```python
from build123d import *

# Parameters (mm, degrees)
BOX007_W          = 10
BOX007_H          = 10
BOX007_DEPTH      = 17
CYLINDER002_R     = 3.4
CYLINDER002_DEPTH = 13
BOX006_W          = 6
BOX006_H          = 10
BOX006_DEPTH      = 15
BOX005_W          = 6
BOX005_H          = 10
BOX005_DEPTH      = 15
CYLINDER001_R     = 15
CYLINDER001_DEPTH = 2.5
BOX004_W          = 6
BOX004_H          = 10
BOX004_DEPTH      = 15
BOX003_W          = 6
BOX003_H          = 10
BOX003_DEPTH      = 15
BOX002_W          = 6
BOX002_H          = 35
BOX002_DEPTH      = 10
BOX001_W          = 15
BOX001_H          = 35
BOX001_DEPTH      = 10
BOX_W             = 15
BOX_H             = 35
BOX_DEPTH         = 10
CYLINDER_R        = 15
CYLINDER_DEPTH    = 12
FILLET_R          = 4
FILLET001_R       = 1.5
FILLET002_R       = 1.5


with BuildPart() as cubo005:
    # Box007 → Box007 (new body)
    with BuildSketch(Plane(origin=(-5, 2.6, -28), x_dir=(1, 0, 0), z_dir=(0, 0, 1))):
        with Locations((5, 5)):
            Rectangle(BOX007_W, BOX007_H)
    extrude(amount=BOX007_DEPTH)


with BuildPart() as cut007:
    # Cylinder002 → Cylinder002 (new body)
    with BuildSketch(Plane.XY.offset(-26)):
        Circle(CYLINDER002_R)
    extrude(amount=CYLINDER002_DEPTH)

    # Cut007: cut Cubo005
    add(cubo005.part, mode=Mode.SUBTRACT)


with BuildPart() as cut007_1:
    # Cut007 placement: moved
    add(cut007.part.moved(Location((0, 0, 23))))


with BuildPart() as cubo004:
    # Box006 → Box006 (new body)
    with BuildSketch(Plane(origin=(-3, 14.4, -2), x_dir=(1, 0, 0), z_dir=(0, 0, 1))):
        with Locations((3, 5)):
            Rectangle(BOX006_W, BOX006_H)
    extrude(amount=BOX006_DEPTH)


with BuildPart() as cubo003:
    # Box005 → Box005 (new body)
    with BuildSketch(Plane(origin=(-3, -24.4, -2), x_dir=(1, 0, 0), z_dir=(0, 0, 1))):
        with Locations((3, 5)):
            Rectangle(BOX005_W, BOX005_H)
    extrude(amount=BOX005_DEPTH)


with BuildPart() as cilindro001:
    # Cylinder001 → Cylinder001 (new body)
    with BuildSketch(Plane.XY.offset(-2)):
        Circle(CYLINDER001_R)
    extrude(amount=CYLINDER001_DEPTH)


with BuildPart() as cubo002:
    # Box004 → Box004 (new body)
    with BuildSketch(Plane(origin=(-3, -24.4, -2), x_dir=(1, 0, 0), z_dir=(0, 0, 1))):
        with Locations((3, 5)):
            Rectangle(BOX004_W, BOX004_H)
    extrude(amount=BOX004_DEPTH)


with BuildPart() as cubo001:
    # Box003 → Box003 (new body)
    with BuildSketch(Plane(origin=(-3, 14.4, -2), x_dir=(1, 0, 0), z_dir=(0, 0, 1))):
        with Locations((3, 5)):
            Rectangle(BOX003_W, BOX003_H)
    extrude(amount=BOX003_DEPTH)


with BuildPart() as cubo:
    # Box002 → Box002 (new body)
    with BuildSketch(Plane(origin=(-3, -17, 11.7), x_dir=(1, 0, 0), z_dir=(0, 0, 1))):
        with Locations((3, 17.5)):
            Rectangle(BOX002_W, BOX002_H)
    extrude(amount=BOX002_DEPTH)


with BuildPart() as box001:
    # Box001 → Box001 (new body)
    with BuildSketch(Plane(origin=(-20, -15, 3), x_dir=(1, 0, 0), z_dir=(0, 0, 1))):
        with Locations((7.5, 17.5)):
            Rectangle(BOX001_W, BOX001_H)
    extrude(amount=BOX001_DEPTH)


with BuildPart() as box:
    # Box → Box (new body)
    with BuildSketch(Plane(origin=(5, -15, 3), x_dir=(1, 0, 0), z_dir=(0, 0, 1))):
        with Locations((7.5, 17.5)):
            Rectangle(BOX_W, BOX_H)
    extrude(amount=BOX_DEPTH)


with BuildPart() as fuel_knob:
    # Cylinder → Cylinder (new body)
    with BuildSketch(Plane.XY):
        Circle(CYLINDER_R)
    extrude(amount=CYLINDER_DEPTH)

    # Cut: cut Box
    add(box.part, mode=Mode.SUBTRACT)

    # Cut001: cut Box001
    add(box001.part, mode=Mode.SUBTRACT)

    # Cut002: cut Cubo
    add(cubo.part, mode=Mode.SUBTRACT)

    # Cut003: cut Cubo001
    add(cubo001.part, mode=Mode.SUBTRACT)

    # Cut004: cut Cubo002
    add(cubo002.part, mode=Mode.SUBTRACT)

    # Fusion: union Cilindro001
    add(cilindro001.part)

    # Cut005: cut Cubo003
    add(cubo003.part, mode=Mode.SUBTRACT)

    # Cut006: cut Cubo004
    add(cubo004.part, mode=Mode.SUBTRACT)

    # Fillet
    fillet_edges = [fuel_knob.edges().sort_by_distance(p)[0] for p in [
        (0, -14.4, 11.7),
        (0, 14.4, 11.7),
        (-4.009607, -14.454171, 12),
        (-4.009607, 14.454171, 12),
        (4.009607, 14.454171, 12),
        (4.009607, -14.454171, 12),
    ]]
    fillet(fillet_edges, radius=FILLET_R)

    # Fillet001
    fillet001_edges = [fuel_knob.edges().sort_by_distance(p)[0] for p in [
        (-5, 0, 3),
        (5, 0, 3),
    ]]
    fillet(fillet001_edges, radius=FILLET001_R)

    # Fillet002
    fillet002_edges = [fuel_knob.edges().sort_by_distance(p)[0] for p in [
        (-5, 0, 12),
        (5, 0, 12),
    ]]
    fillet(fillet002_edges, radius=FILLET002_R)

    # Cut008: cut Cut007
    add(cut007_1.part, mode=Mode.SUBTRACT)


solid = fuel_knob.part
```
Input: part model. Units: mm. Frame: model coordinates. A direction names the side the tool comes from. Give positions to 0.01 mm unless a question says otherwise; leave off trailing zeros. Write each loop counter-clockwise with the first axis right and the second up, starting at its lowest first coordinate (ties: lowest second). Pieces come first, ordered by that corner, then holes. Notation, with made-up numbers: (7, 39.25) - (37, 39.25) arc R35 ccw to (37, 74.25) - close; hole circle Ø3 at (-4, 2). An arc over 180 degrees is marked (long way). Write item = value, one per line. Start each with the question number.
1. Section query D-D, the plane z = 5.5. Output: boundary loops of the cut face in (x, y), then the cut area to 3 significant figures.
2. Section query C-C, the plane x = 0. Output: boundary loops of the cut face in (y, z), then the cut area to 3 significant figures.
3. Access query for faces 1 (the flat face through (0, 2.6, 4)), 2 (the flat face through (0, 0, 11.7)), 3 (the cylindrical face through (-4.682, -13.962, 6.226)), 4 (the cylindrical face through (-0.042, -13.197, 10.559)), 5 (the flat face through (5, 0, 7)). Directions: +Z, -Z, +X, -X, +Y, -Y. A direction counts if a zero-diameter tool reaches every point of the face in a straight line with its end or side. Return the directions, or none.
4. First-contact query: pin 1 Ø8 at (x, z) = (-8.5, 0.5) entering from -Y; pin 2 Ø7.5 at (x, y) = (-10.5, -5) entering from +Z; pin 3 Ø2 at (y, z) = (-7, 8) entering from -X; pin 4 Ø11 at (x, y) = (0, 0) entering from +Z. Flat tips, straight axial feed; report the tip coordinate or a pass-through.
5. Section query B-B, the plane y = 0. Output: boundary loops of the cut face in (x, z), then the cut area to 3 significant figures.
6. Ray query, L1, parallel to X at y = 0, z = 4.75; L2, parallel to Y at x = 0, z = 5.75; L3, parallel to Z at x = 12, y = 3.25. Return the intervals inside material, ascending.
7. Section query A-A, the plane z = 1. Output: boundary loops of the cut face in (x, y), then the cut area to 3 significant figures.
Check sheet entries:
q1.outline = (-5, -13.04) arc R1.5 ccw to (-3.89, -14.49) arc R15 ccw to (-3, -14.7) - (-3, -14.4) - (3, -14.4) - (3, -14.7) arc R15 ccw to (3.89, -14.49) arc R1.5 ccw to (5, -13.04) - (5, 13.04) arc R1.5 ccw to (3.89, 14.49) arc R15 ccw to (3, 14.7) - (3, 14.4) - (-3, 14.4) - (-3, 14.7) arc R15 ccw to (-3.89, 14.49) arc R1.5 ccw to (-5, 13.04) - close; hole (-2.19, 2.6) arc R3.4 ccw (long way) to (2.19, 2.6) - close
q1.area = 253 mm2
q2.outline = (-14.4, -2) - (-3.4, -2) - (-3.4, 10) - (2.6, 10) - (2.6, -2) - (14.4, -2) - (14.4, 7.7) arc R4 ccw to (10.4, 11.7) - (-10.4, 11.7) arc R4 ccw to (-14.4, 7.7) - close
q2.area = 316 mm2
q3.face_1 = -Z
q3.face_2 = +Z, +Y, -Y
q3.face_3 = +Z, -X, -Y
q3.face_4 = +Z, -Y
q3.face_5 = +Z, +X, +Y, -Y
q4.pin_1 = -14.31
q4.pin_2 = 3
q4.pin_3 = -5
q4.pin_4 = 12
q5.outline = (-15, -2) - (-3.4, -2) - (-3.4, 10) - (3.4, 10) - (3.4, -2) - (15, -2) - (15, 1.5) arc R1.5 ccw to (13.5, 3) - (6.5, 3) arc R1.5 cw to (5, 4.5) - (5, 10.5) arc R1.5 ccw to (3.5, 12) - (3, 12) - (3, 11.7) - (-3, 11.7) - (-3, 12) - (-3.5, 12) arc R1.5 ccw to (-5, 10.5) - (-5, 4.5) arc R1.5 cw to (-6.5, 3) - (-13.5, 3) arc R1.5 ccw to (-15, 1.5) - close
q5.area = 156 mm2
q6.L1 = -5 to -3.4, 3.4 to 5
q6.L2 = -14.4 to -3.4, 2.6 to 14.4
q6.L3 = -2 to 3
q7.outline = (-3, -14.7) - (-3, -14.4) - (3, -14.4) - (3, -14.7) arc R15 ccw to (3, 14.7) - (3, 14.4) - (-3, 14.4) - (-3, 14.7) arc R15 ccw to start; hole (-2.19, 2.6) arc R3.4 ccw (long way) to (2.19, 2.6) - close
q7.area = 667 mm2
